Autodesk Inventor part; units mm, degrees
ref_plane "YZ Plane" through (0, 0, 0) normal (1, 0, 0) x (0, 1, 0)
ref_plane "XZ Plane" through (0, 0, 0) normal (0, 1, 0) x (-1, 0, 0)
ref_plane "XY Plane" through (0, 0, 0) normal (0, 0, 1) x (1, 0, 0)
sketch "Boceto1" plane through (0, 0, 0) normal (0, 0, 1) x (1, 0, 0)
  circle A0 centre (0, 23.4183) radius 11
  circle A1 centre (0, 23.4183) radius 16
  line L0 (-16, 23.4183) -> (-16, -2.7)
  line L1 (16, 23.4183) -> (16, -2.7)
  line L2 (-25, 0.1183) -> (25, 0.1183)
  line L3 (25, 0.1183) -> (25, 10.1183)
  line L4 (25, 10.1183) -> (-25, 10.1183)
  line L5 (-25, 10.1183) -> (-25, 0.1183)
  point P0 (0, 0)
  point P1 (0, 0.1183)
  point P2 (-16, 10.1183)
  point P3 (16, 10.1183)
  dimension "d0" = 22
  dimension "d1" = 32
  dimension "d2" = 50
  dimension "d11" = 10
  dimension "d23" = 23.3
extrude "Extrusión1" add sketch "Boceto1" along normal blind 20 contours L4 L1 L2 L0 A1 | A1 L4 | L4 L3 L2 L1 | L0 L2 L5 L4 picked at (-1.8471, 9.5484)
extrude "Extrusión2" add sketch "Boceto1" along normal blind 15 contours A1 L4 | L1 L4 A1 | A1 L4 L0 picked at (0.442, 10.9117)
sketch "Boceto3" plane through (-25, 0.1183, 0) normal (0, -1, 0) x (1, 0, 0)
  line L0 (0, 20) -> (50, 20)
  line L1 (7.5, 20) -> (42.5, 20)
  line L2 (42.5, 20) -> (42.5, 0)
  line L3 (42.5, 0) -> (7.5, 0)
  line L4 (7.5, 0) -> (7.5, 20)
  line L5 (0, 0) -> (50, 0)
  line L6 (0, 0) -> (50, 0)
  line L7 (50, 0) -> (50, 20)
  line L8 (0, 20) -> (50, 20)
  line L9 (0, 0) -> (0, 20)
  point P0 (25, 0)
  point P1 (25, 20)
  point P2 (25, 0)
  dimension "d8" = 35
extrude "Extrusión3" add sketch "Boceto3" along normal blind 20 contours L0 L4 L5 L9 | L0 L7 L5 L2
sketch "Boceto4" plane through (-25, 10.1183, 0) normal (-1, 0, 0) x (0, 0, 1)
  line L0 (0, -10.1183) -> (0, -30)
  line L1 (0, -30) -> (20, -30)
  line L2 (0, -20) -> (20, -20)
  line L3 (20, -20) -> (20, -30)
  line L4 (20, -30) -> (0, -30)
  line L5 (0, -30) -> (0, -20)
  dimension "d12" = 10
extrude "Extrusión4" add sketch "Boceto4" along normal blind 15
mirror "Simetría1" about plane through (0, 0, 0) normal (1, 0, 0) of "Extrusión4"
sketch "Boceto5" plane through (-25, -9.8817, 20) normal (0, 1, 0) x (1, 0, 0)
  circle A0 centre (-9, 15) radius 1.9844
  circle A1 centre (-9, 5) radius 1.9844
  line L0 (0, 20) -> (-15, 20)
  line L1 (0, 0) -> (-15, 0)
  line L2 (-15, 0) -> (-15, 20)
  point P0 (25, 20)
  dimension "d15" = 3.9688
  dimension "d16" = 3.9688
  dimension "d17" = 5
  dimension "d18" = 5
  dimension "d19" = 6
  dimension "d20" = 6
extrude "Extrusión5" cut sketch "Boceto5" against normal through all
mirror "Simetría2" about plane through (0, 0, 0) normal (1, 0, 0) of "Extrusión5"
properties part number "soporte_balineras"
CAD build for the part. Positions are in the model's coordinates, mm. A direction names the side the tool comes from. Give positions to 0.01 mm unless a question says otherwise; leave off trailing zeros. Loops run counter-clockwise (first coordinate to the right, second up) from the corner with the lowest first, then second, coordinate; pieces in that order, holes last. Notation, with made-up numbers: M 88,19.5 L 108,19.5 A15 cw 108,47.5 Z; hole C 83.25,77 d9. An arc over 180 degrees is marked long. Write each question's results on one line, items separated by ' | '.
Q1. Band-saw the part on A-A on z = 5. Write the cut outline in (x, y).
Geometry check:
outline: M -40,-19.88 L -35.98,-19.88 L -35.98,-9.88 L -40,-9.88 Z; M -32.02,-19.88 L -17.5,-19.88 L -17.5,0.12 L 17.5,0.12 L 17.5,-19.88 L 32.02,-19.88 L 32.02,-9.88 L 25,-9.88 L 25,10.12 L 16,10.12 L 16,23.42 A16 ccw -16,23.42 L -16,10.12 L -25,10.12 L -25,-9.88 L -32.02,-9.88 Z; M 35.98,-19.88 L 40,-19.88 L 40,-9.88 L 35.98,-9.88 Z; hole C 0,23.42 d22
Q2. Probe probe 1 along X at (y, z) = (-12.75, 5); probe 2 along Z at (x, y) = (34, -10); probe 3 along Y at (x, z) = (0, 6.5). List the from-to ranges inside material, lowest first.
Geometry check:
probe 1: x = -40 to -35.98, -32.02 to -17.5, 17.5 to 32.02, 35.98 to 40 | probe 2: z = 0 to 3.02, 6.98 to 13.02, 16.98 to 20 | probe 3: y = 0.12 to 12.42, 34.42 to 39.42
Q3. Flat gauge pins, fed straight in: P1, Ø3, axis at x = -34, z = 15, coming from the -Y side; P2, Ø4, axis at y = 16, z = 10.5, coming from the -X side; P3, Ø6, axis at y = 17.5, z = 12, coming from the +X side; P4, Ø4.5, axis at x = -34, z = 5, coming from the +Y side. Where does each tip first touch, or does it go through?
Geometry check:
P1: passes through | P2: stops at x = -16 | P3: stops at x = 16 | P4: stops at y = -9.88
Q4. Band-saw the part on C-C on z = 9.25. Write the cut outline in (x, y).
Geometry check:
outline: M -40,-19.88 L -17.5,-19.88 L -17.5,0.12 L 17.5,0.12 L 17.5,-19.88 L 40,-19.88 L 40,-9.88 L 25,-9.88 L 25,10.12 L 16,10.12 L 16,23.42 A16 ccw -16,23.42 L -16,10.12 L -25,10.12 L -25,-9.88 L -40,-9.88 Z; hole C 0,23.42 d22
Q5. Mould opens along Z. For faces 6 (the face through (16, 17, 7)), 7 (the face through (-32.167, -14.812, 15.76)), 8 (the face through (-11, 18, 15)) say: pulls with the +Z half, pulls with the -Z half, needs draft (parallel to the pull), parting line crosses it, or undercut.
Geometry check:
face 6: needs draft | face 7: undercut | face 8: pulls with the +Z half
Q6. Band-saw the part on D-D on x = 7. Write the cut outline in (y, z).
Geometry check:
outline: M 0.12,0 L 14.93,0 L 14.93,15 L 10.12,15 L 10.12,20 L 0.12,20 Z; M 31.9,0 L 37.81,0 L 37.81,15 L 31.9,15 Z
Q7. Which spindle directions (+Z, -Z, +X, -X, +Y, -Y) get a long thin tool onto all of the face, cutting with end or side? Do faces 1 (the face through (32, -9.882, 10)), 2 (the face through (0, 0.118, 10)), 3 (the face through (-32.167, -14.812, 5.76)), 4 (the face through (-32, -9.882, 10)), 5 (the face through (-29, -19.882, 10)). Say none if no direction does.
Geometry check:
face 1: +Z, -Z, +X, +Y | face 2: +Z, -Z, -Y | face 3: +Y, -Y | face 4: +Z, -Z, -X, +Y | face 5: +Z, -Z, +X, -X, -Y
Q8. Band-saw the part on B-B on x = -34. Write the cut outline in (y, z), and give its area (3 significant figures).
Geometry check:
outline: M -19.88,0 L -9.88,0 L -9.88,3.02 L -19.88,3.02 Z; M -19.88,6.98 L -9.88,6.98 L -9.88,13.02 L -19.88,13.02 Z; M -19.88,16.98 L -9.88,16.98 L -9.88,20 L -19.88,20 Z | area: 121 mm²
